Autodesk Inventor part; units mm, degrees
ref_plane "YZ Plane" through (0, 0, 0) normal (1, 0, 0) x (0, 1, 0)
ref_plane "XZ Plane" through (0, 0, 0) normal (0, 1, 0) x (-1, 0, 0)
ref_plane "XY Plane" through (0, 0, 0) normal (0, 0, 1) x (1, 0, 0)
sketch "Sketch1" plane through (0, 0, 0) normal (0, 1, 0) x (-1, 0, 0)
  line L0 (0, 0) -> (248, 0)
  line L1 (248, 0) -> (248, -75)
  line L2 (248, -75) -> (0, -75)
  line L3 (0, -75) -> (0, 0)
  dimension "d0" = 248
  dimension "d1" = 75
extrude "Extrusion1" add sketch "Sketch1" along normal blind 50.8
sketch "Sketch2" plane through (0, 50.8, 0) normal (0, 1, 0) x (1, 0, 0)
  circle A0 centre (-196, 65) radius 7.5
  line L0 (0, 75) -> (-248, 75)
  line L1 (-248, 75) -> (-248, 0)
  circle A1 centre (-154, 65) radius 7.5
  circle A2 centre (-112, 65) radius 7.5
  circle A3 centre (-70, 65) radius 7.5
  point P0 (0, 0)
  dimension "d4" = 15
  dimension "d5" = 10
  dimension "d6" = 52
  dimension "d12" = 42
extrude "Extrusion2" cut sketch "Sketch2" against normal blind 50.8
sketch "Sketch3" plane through (0, 50.8, 0) normal (0, 1, 0) x (1, 0, 0)
  line L0 (0, 75) -> (-248, 75)
  line L1 (-198.5, 75) -> (-193.5, 75)
  line L2 (-193.5, 75) -> (-193.5, 72)
  line L3 (-193.5, 72) -> (-198.5, 72)
  line L4 (-198.5, 72) -> (-198.5, 75)
  circle A0 centre (-196, 65) radius 7.5
  line L5 (-151.5, 75) -> (-151.5, 72)
  line L6 (-151.5, 72) -> (-156.5, 72)
  line L7 (-156.5, 72) -> (-156.5, 75)
  line L8 (-156.5, 75) -> (-151.5, 75)
  line L9 (-109.5, 75) -> (-109.5, 72)
  line L10 (-109.5, 72) -> (-114.5, 72)
  line L11 (-114.5, 72) -> (-114.5, 75)
  line L12 (-114.5, 75) -> (-109.5, 75)
  line L13 (-67.5, 75) -> (-67.5, 72)
  line L14 (-67.5, 72) -> (-72.5, 72)
  line L15 (-72.5, 72) -> (-72.5, 75)
  line L16 (-72.5, 75) -> (-67.5, 75)
  point P0 (0, 0)
  dimension "d16" = 5
  dimension "d17" = 3
  dimension "d18" = 2.5
  dimension "d24" = 42
extrude "Extrusion3" cut sketch "Sketch3" against normal blind 50.8 contours L13 L14 L15 L0 | L2 A0 L4 L0 | L5 L6 L7 L0 | L9 L10 L11 L0 | L2 L3 L4 A0 picked at (-196.2826, 72.1506)
properties part number "Lateral"
CAD build for the part. Positions are in the model's coordinates, mm. Round coordinates to 2 decimals unless told otherwise and drop trailing zeros. Order: outer loops, then holes, each group sorted by start corner. A loop starts at its lowest first (then second) coordinate and runs counter-clockwise, first axis right, second up.
Q1. Slice it at D-D (x = -70). Write the cut outline in (y, z).
Q2. Wall check: L1, parallel to X at y = 20, z = -65; L2, parallel to X at y = 31, z = -71.5; L3, parallel to Z at x = -70, y = 3.5. Give the ranges that are in metal, low to high.
Q3. Slice it at C-C (x = -117). Write the cut outline in (y, z).
Q4. Slice it at B-B (y = 19). Write the cut outline in (x, z), and give its area (3 significant figures).
Q5. Two-plate mould, pull along Z, no slides. Class faces 1 (the flat face through (-91, 25, -75)), 2 (the cylindrical face through (-154.294, 25.756, -57.506)), 3 (the flat face through (-248, 25, -37)): pulls with the +Z half, pulls with the -Z half, needs draft (parallel to the pull), parting line crosses it, or undercut.
Q6. Slice it at A-A (z = -62.5). Write the cut outline in (x, y).
Results below:
1. outline: (0, -57.5) - (50.8, -57.5) - (50.8, 0) - (0, 0) - close
2. L1: x = -248 to -203.5, -188.5 to -161.5, -146.5 to -119.5, -104.5 to -77.5, -62.5 to 0
2. L2: x = -248 to -199.74, -192.26 to -157.74, -150.26 to -115.74, -108.26 to -73.74, -66.26 to 0
2. L3: z = -57.5 to 0
3. outline: (0, -75) - (50.8, -75) - (50.8, -70.59) - (0, -70.59) - close; (0, -59.41) - (50.8, -59.41) - (50.8, 0) - (0, 0) - close
4. outline: (-248, -75) - (-198.5, -75) - (-198.5, -72.07) arc R7.5 cw (long way) to (-193.5, -72.07) - (-193.5, -75) - (-156.5, -75) - (-156.5, -72.07) arc R7.5 cw (long way) to (-151.5, -72.07) - (-151.5, -75) - (-114.5, -75) - (-114.5, -72.07) arc R7.5 cw (long way) to (-109.5, -72.07) - (-109.5, -75) - (-72.5, -75) - (-72.5, -72.07) arc R7.5 cw (long way) to (-67.5, -72.07) - (-67.5, -75) - (0, -75) - (0, 0) - (-248, 0) - close
4. area: 17,800 mm2
5. face 1: pulls with the -Z half
5. face 2: undercut
5. face 3: needs draft
6. outline: (-248, 0) - (-203.07, 0) - (-203.07, 50.8) - (-248, 50.8) - close; (-188.93, 0) - (-161.07, 0) - (-161.07, 50.8) - (-188.93, 50.8) - close; (-146.93, 0) - (-119.07, 0) - (-119.07, 50.8) - (-146.93, 50.8) - close; (-104.93, 0) - (-77.07, 0) - (-77.07, 50.8) - (-104.93, 50.8) - close; (-62.93, 0) - (0, 0) - (0, 50.8) - (-62.93, 50.8) - close
